```python
from build123d import *

# Parameters (mm, degrees)
F0_R     = 2.55
F1_DEPTH = 6
F3_DEPTH = 3
F6_DEPTH = 1.2


with BuildPart() as f1:
    # F0 (on Top) → F1 (new body)
    with BuildSketch(Plane.XY):
        with BuildLine():
            ThreePointArc((-31.0288725662, 20.2239290055), (-32.9870436526, 22.0241242247), (-33.9929573966, 24.4864959209))
            ThreePointArc((-33.9929573966, 24.4864959209), (-43.8, 29.0984535672), (-44.7094488189, 18.2993267135))
            ThreePointArc((-44.7094488189, 18.2993267135), (-43.0799292484, 16.196994009), (-42.5, 13.6010704937))
            Line((-42.5, 13.6010704937), (-42.5, -13.6010704937))
            ThreePointArc((-42.5, -13.6010704937), (-43.0799292484, -16.196994009), (-44.7094488189, -18.2993267135))
            ThreePointArc((-44.7094488189, -18.2993267135), (-43.8, -29.0984535672), (-33.9929573966, -24.4864959209))
            ThreePointArc((-33.9929573966, -24.4864959209), (-32.9870429643, -22.0241232349), (-31.0288704781, -20.2239277999))
            Line((-31.0288704781, -20.2239277999), (-21.8480739571, -14.9233924572))
            ThreePointArc((-21.8480739571, -14.9233924572), (-21.1160231495, -12.1913416496), (-23.8480739571, -11.459290842))
            Line((-23.8480739571, -11.459290842), (-33.0288704781, -16.7598261848))
            ThreePointArc((-33.0288704781, -16.7598261848), (-36.6762898114, -16.7598279931), (-38.5, -13.6010704937))
            Line((-38.5, -13.6010704937), (-38.5, 13.6010704937))
            ThreePointArc((-38.5, 13.6010704937), (-36.6762908554, 16.7598273904), (-33.0288725662, 16.7598273904))
            Line((-33.0288725662, 16.7598273904), (-9.4711274338, 3.1587568967))
            ThreePointArc((-9.4711274338, 3.1587568967), (-7.6474182892, 6.361e-07), (-9.471126332, -3.1587562606))
            Line((-9.471126332, -3.1587562606), (-18.6519224918, -8.4592913948))
            ThreePointArc((-18.6519224918, -8.4592913948), (-19.383972999, -11.1913405115), (-16.6519239586, -11.9233913037))
            Line((-16.6519239586, -11.9233913037), (-7.471126332, -6.6228578757))
            ThreePointArc((-7.471126332, -6.6228578757), (-4.9330264651, -5.8271301623), (-2.2975937845, -6.1871692074))
            ThreePointArc((-2.2975937845, -6.1871692074), (6.6, 0), (-2.2975937845, 6.1871692074))
            ThreePointArc((-2.2975937845, 6.1871692074), (-4.933027099, 5.8271302157), (-7.4711274338, 6.6228585118))
            Line((-7.4711274338, 6.6228585118), (-31.0288725662, 20.2239290055))
        make_face()
        with Locations((-40.5, -23.3826859022)):
            Circle(F0_R, mode=Mode.SUBTRACT)
        Circle(F0_R, mode=Mode.SUBTRACT)
        with Locations((-40.5, 23.3826859022)):
            Circle(F0_R, mode=Mode.SUBTRACT)
    extrude(amount=F1_DEPTH)

    # F2 (on face) → F3 (cut)
    with BuildSketch(Plane.XY.offset(6)):
        Polygon((-36.55, 21.1021523389), (-36.55, 25.6632194655), (-40.5, 27.9437530288), (-44.45, 25.6632194655), (-44.45, 21.1021523389), (-40.5, 18.8216187756), align=None)
        Polygon((-36.55, -25.6632194655), (-36.55, -21.1021523389), (-40.5, -18.8216187756), (-44.45, -21.1021523389), (-44.45, -25.6632194655), (-40.5, -27.9437530288), align=None)
        Polygon((-3.95, 2.2805335633), (-3.95, -2.2805335633), (0, -4.5610671266), (3.95, -2.2805335633), (3.95, 2.2805335633), (0, 4.5610671266), align=None)
    extrude(amount=-F3_DEPTH, mode=Mode.SUBTRACT)

    # F5 (on mid) → F6 (cut, symmetric)
    with BuildSketch(Plane.XY.offset(3)):
        with BuildLine():
            Line((-23.8480739571, -11.459290842), (-25.8992931068, -12.6435627702))
            ThreePointArc((-25.8992931068, -12.6435627702), (-25.5327527088, -14.7413416496), (-23.8992931068, -16.1076643854))
            Line((-23.8992931068, -16.1076643854), (-21.8480739571, -14.9233924572))
            ThreePointArc((-21.8480739571, -14.9233924572), (-24.5801247646, -14.1913416496), (-23.8480739571, -11.459290842))
        make_face()
        with BuildLine():
            ThreePointArc((-18.6519224918, -8.4592913948), (-15.9198730901, -9.1913419783), (-16.6519239586, -11.9233913037))
            Line((-16.6519239586, -11.9233913037), (-14.6007037534, -10.7391193365))
            ThreePointArc((-14.6007037534, -10.7391193365), (-14.9672441312, -8.6413415249), (-16.6007025337, -7.2750189998))
            Line((-16.6007025337, -7.2750189998), (-18.6519224918, -8.4592913948))
        make_face()
    extrude(amount=F6_DEPTH, both=True, mode=Mode.SUBTRACT)


solid = f1.part
```
The model under review builds one solid part; all positions refer to its coordinate system, in mm. A direction names the side the tool comes from. Coordinates: 2 decimals unless noted, no trailing zeros. Write each loop counter-clockwise with the first axis right and the second up, starting at its lowest first coordinate (ties: lowest second). Pieces come first, ordered by that corner, then holes. Notation, with made-up numbers: (45, 85) - (104, 85) arc R31 cw to (104, 122) - close; hole circle Ø9 at (7, -18.75). An arc over 180 degrees is marked (long way). Answer in a Markdown table with one row per item. Add a question column.
Q1. Consider section C-C on x = -8.5. Give the boundary of the cut face in (y, z).
Q2. For faces 1 (the face through (-15.7, -9.1, 4.2)), 2 (the face through (-38.553, 19.946, 4.521)), 3 (the face through (-21.41, 10.05, 2.96)), list the 3-axis set-ups (+Z, -Z, +X, -X, +Y, -Y) from which the entire face can be reached by the end or side of a thin tool; tool diameter is ignored.
Q3. Clearance check with flat-ended pins moving along their axes: pin 1 (4 mm diameter, centred on x = -32.5, y = 13, fed in from +Z); pin 2 (0.9 mm diameter, centred on y = -24, z = 4.5, fed in from +X); pin 3 (1.5 mm diameter, centred on y = 13, z = 5, fed in from +X); pin 4 (0.9 mm diameter, centred on y = 1, z = 5, fed in from +X). State where each tip first meets the part, or that it passes through.
Q4. Consider section A-A on y = -9.5. Give the boundary of the cut face in (x, z), then the cut area to 3 significant figures.
Q5. Consider section B-B on y = 0. Give the boundary of the cut face in (x, z), then the cut area to 3 significant figures.
Q6. To check wall thickness, follow line 1 along Y through (x, z) = (-40.5, 1.2); line 2 along X through (y, z) = (-3, 2.55); line 3 along Y through (x, z) = (-21.5, 3.6). State the ranges of each line that lie inside material, in increasing order. Write a range as from..to.
Q7. Draft analysis for pull direction X (two halves, no side actions). For faces 4 (the face through (-43.64, 29.19, 2.96)), 5 (the face through (-38.55, -26.82, 4.52)), 6 (the face through (-26.5, -17.61, 2.96)), state which applies: +X half, -X half, draft (parallel to the pull), parting line (faces both ways), or undercut.
Q8. Consider section D-D on z = 0.85. Give the boundary of the cut face in (x, y).
Answers below:
| question | item | result |
|---|---|---|
| 1 | outline | (-7.22, 0) - (-2.34, 0) - (-2.34, 6) - (-7.22, 6) - close; (2.34, 0) - (7.22, 0) - (7.22, 6) - (2.34, 6) - close |
| 2 | face 1 | none |
| 2 | face 2 | +Z |
| 2 | face 3 | +Z, -Z |
| 3 | pin 1 | through |
| 3 | pin 2 | x = -33.76 |
| 3 | pin 3 | x = -17.22 |
| 3 | pin 4 | x = 6.58 |
| 4 | outline | (-42.5, 0) - (-38.5, 0) - (-38.5, 6) - (-42.5, 6) - close; (-19.53, 0) - (-12.45, 0) - (-12.45, 6) - (-19.53, 6) - close; hole (-15.78, 1.8) - (-14.63, 1.8) - (-14.63, 4.2) - (-15.78, 4.2) - close |
| 4 | area | 63.7 mm² |
| 5 | outline | (-42.5, 0) - (-38.5, 0) - (-38.5, 6) - (-42.5, 6) - close; (-7.65, 0) - (-2.55, 0) - (-2.55, 3) - (-3.95, 3) - (-3.95, 6) - (-7.65, 6) - close; (2.55, 0) - (6.6, 0) - (6.6, 6) - (3.95, 6) - (3.95, 3) - (2.55, 3) - close |
| 5 | area | 70.5 mm² |
| 6 | line 1 | -29.98..-25.93, -20.83..20.83, 25.93..29.98 |
| 6 | line 2 | -42.5..-38.5, -9.22..5.88 |
| 6 | line 3 | -14.67..-11.71, 10.1..14.72 |
| 7 | face 4 | parting line |
| 7 | face 5 | undercut |
| 7 | face 6 | +X half |
| 8 | outline | (-44.71, -18.3) arc R6.6 ccw (long way) to (-33.99, -24.49) arc R6.1 cw to (-31.03, -20.22) - (-21.85, -14.92) arc R2 ccw to (-23.85, -11.46) - (-33.03, -16.76) arc R3.65 cw to (-38.5, -13.6) - (-38.5, 13.6) arc R3.65 cw to (-33.03, 16.76) - (-9.47, 3.16) arc R3.65 cw to (-9.47, -3.16) - (-18.65, -8.46) arc R2 ccw to (-16.65, -11.92) - (-7.47, -6.62) arc R6.1 cw to (-2.3, -6.19) arc R6.6 ccw (long way) to (-2.3, 6.19) arc R6.1 cw to (-7.47, 6.62) - (-31.03, 20.22) arc R6.1 cw to (-33.99, 24.49) arc R6.6 ccw (long way) to (-44.71, 18.3) arc R6.1 cw to (-42.5, 13.6) - (-42.5, -13.6) arc R6.1 cw to start; hole circle Ø5.1 at (-40.5, -23.38); hole circle Ø5.1 at (-40.5, 23.38); hole circle Ø5.1 at (0, 0) |
